Here's the drawing with two shaded views (mm, measured from the low corner). I have some questions. Give positions to 0.01 mm unless a question says otherwise; leave off trailing zeros. Order: outer loops, then holes, each group sorted by start corner. A loop starts at its lowest first (then second) coordinate and runs counter-clockwise, first axis right, second up. Notation, with made-up numbers: M 29.5,81 L 37.5,81 A33 ccw 37.5,118 Z; hole C -20.75,33.5 d6. An arc over 180 degrees is marked long. Write each question's results on one line, items separated by ' | '.
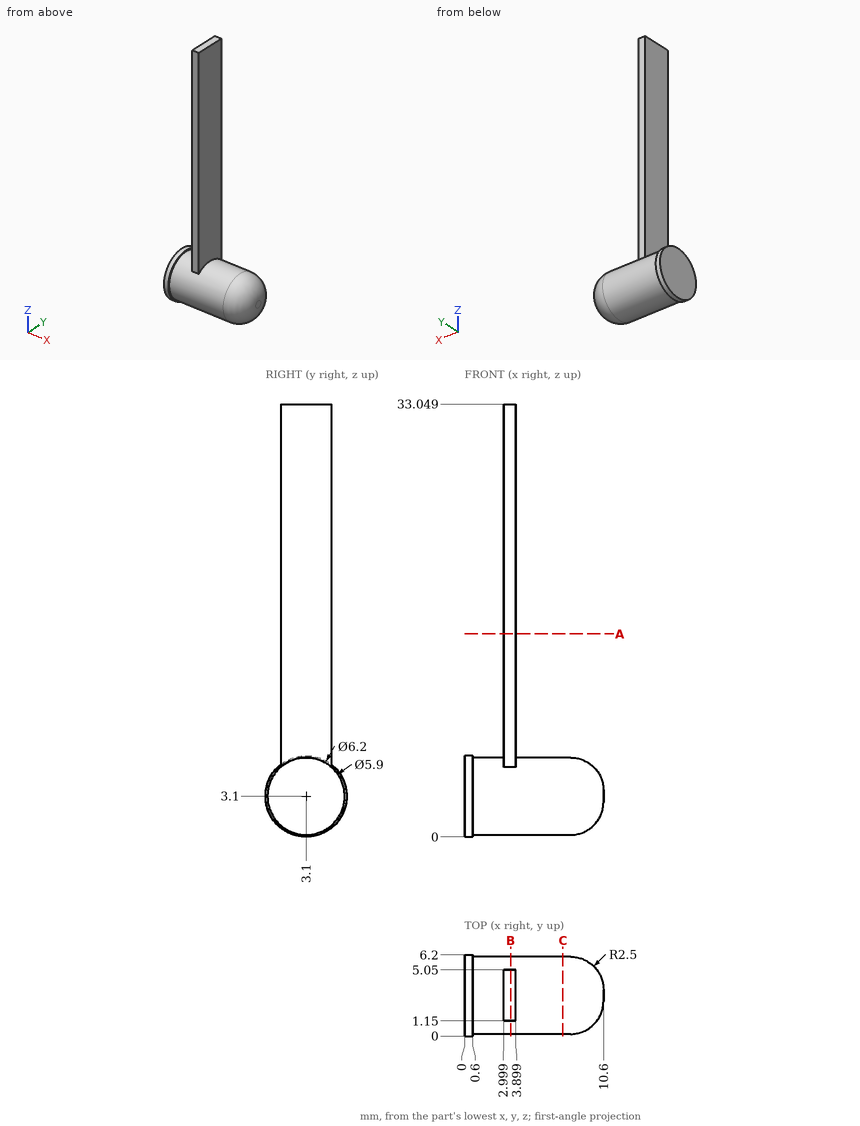
(1) Imagine slicing it at B-B, the plane x = 3.5. Write out the boundary of the cut face in (y, z).
Data:
outline: M 1.15,5.31 A2.95 ccw long 5.05,5.31 L 5.05,33.05 L 1.15,33.05 Z
(2) Imagine slicing it at C-C, the plane x = 7.5. Write out the boundary of the cut face in (y, z).
Data:
outline: C 3.1,3.1 d5.9
(3) I need wall thicknesses on L1, parallel to X at y = 3.5, z = 27; L2, parallel to Y at x = 3.75, z = 24; L3, parallel to Y at x = 1.5, z = 2. Which ranges of each line are inside material? Lowest first, please. Write a range as from..to.
Data:
L1: x = 3..3.9 | L2: y = 1.15..5.05 | L3: y = 0.36..5.84
(4) Imagine slicing it at A-A, the plane z = 15.5. Write out the boundary of the cut face in (x, y).
Data:
outline: M 3,1.15 L 3.9,1.15 L 3.9,5.05 L 3,5.05 Z
(5) Will these pins go through, and if not, where does the flat tip stop? P1, Ø2, axis at y = 4, z = 21.5, coming from the -X side; P2, Ø1.9, axis at y = 3.5, z = 4, coming from the +X side; P3, Ø2, axis at y = 3.5, z = 8.5, coming from the +X side; P4, Ø6, axis at x = 4, z = 16, coming from the -Y side.
Data:
P1: stops at x = 3 | P2: stops at x = 10.6 | P3: stops at x = 3.9 | P4: stops at y = 1.15
